Part print with two shaded views. Sizes in mm from the minimum x, y, z corner. A direction names the side the tool comes from. Round coordinates to 2 decimals unless told otherwise and drop trailing zeros. Write each loop counter-clockwise with the first axis right and the second up, starting at its lowest first coordinate (ties: lowest second). Pieces come first, ordered by that corner, then holes. Notation, with made-up numbers: (71, 85.5) -> (91, 85.5) arc R30 ccw to (91, 109.5) -> close; hole circle Ø7 at (32.25, 13). An arc over 180 degrees is marked (long way). Return JSON: item names as keys, results as strings. Group by question number.
(1) Drop flat-ended pins along their axis: pin 1 Ø2 at (x, y) = (6.5, 7.5) entering from +Z; pin 2 Ø1.5 at (x, y) = (18.5, 12.5) entering from -Z; pin 3 Ø2 at (y, z) = (14, 13) entering from +X. Give the stop position or say it passes through.
(2) Saw through at D-D (y = 2). List the corners of the cut face in (x, z), plus the area to 3 significant figures.
(3) Saw through at A-A (y = 13.75). List the corners of the cut face in (x, z).
(4) Mould opens along X. For the marked faces 3, 4 and 5 say: +X half, -X half, draft (parallel to the pull), parting line (faces both ways), or undercut.
(5) Saw through at B-B (z = 15.5). List the corners of the cut face in (x, y).
(6) Saw through at C-C (x = 15.5). List the corners of the cut face in (y, z), plus the area to 3 significant figures.
(7) Drill centre lines: L1, parallel to Y at x = 8.5, z = 6; L2, parallel to X at y = 13.5, z = 13; L3, parallel to X at y = 15.75, z = 25. Where is each one in solid material? Low to high. Write a range as from..to.
(8) Tool access for the marked faces 1 and 2: list every direction of +Z, -Z, +X, -X, +Y, -Y with a clear straight run to the whole face (end or side of a thin tool).
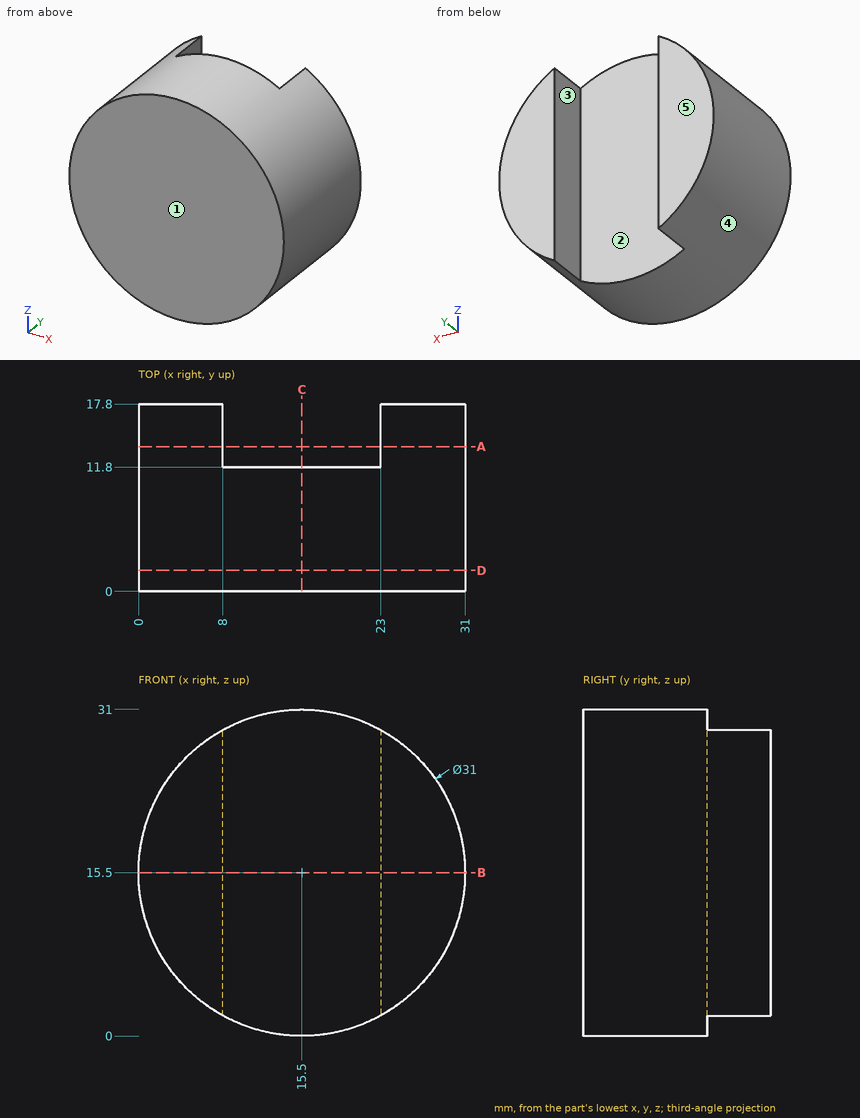
Computed values:
{
 "1": {"pin 1": "z = 28.78", "pin 2": "z = 0.24", "pin 3": "x = 30.93"},
 "2": {"outline": "circle Ø31 at (15.5, 15.5)", "area": "755 mm2"},
 "3": {"outline": "(8, 1.94) -> (8, 29.06) arc R15.5 ccw to start; (23, 1.94) arc R15.5 ccw to (23, 29.06) -> close"},
 "4": {"face 3": "undercut", "face 4": "parting line", "face 5": "draft"},
 "5": {"outline": "(0, 0) -> (31, 0) -> (31, 17.8) -> (23, 17.8) -> (23, 11.8) -> (8, 11.8) -> (8, 17.8) -> (0, 17.8) -> close"},
 "6": {"outline": "(0, 0) -> (11.8, 0) -> (11.8, 31) -> (0, 31) -> close", "area": "366 mm2"},
 "7": {"L1": "0..11.8", "L2": "0.2..8, 23..30.8", "L3": "3.25..8, 23..27.75"},
 "8": {"face 1": "+Z, -Z, +X, -X, -Y", "face 2": "+Z, -Z, +Y"}
}
